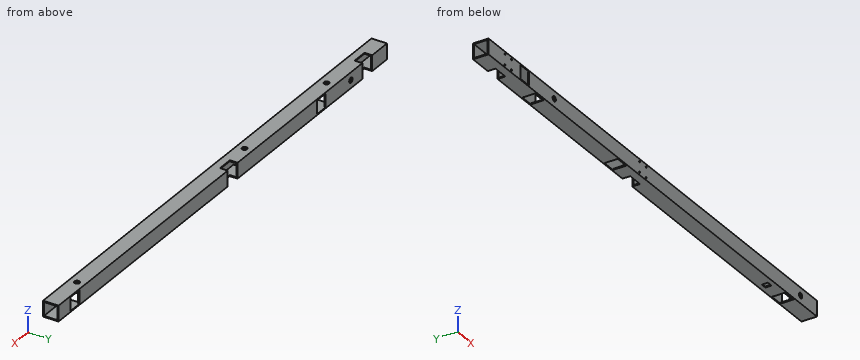
from build123d import *

# Parameters (mm, degrees)
SKETCH_2_W          = 30
SKETCH_2_H          = 30
SKETCH_2_W_2        = 26
SKETCH_2_H_2        = 26
EXTRUDE_2_DEPTH     = 1000
SKETCH_3_W          = 30
SKETCH_3_H          = 15
CUT_EXTRUDE_1_DEPTH = 30
SKETCH_4_W          = 26
SKETCH_4_H          = 26
SKETCH_4_W_2        = 11
SKETCH_4_H_2        = 12
CUT_EXTRUDE_2_DEPTH = 15
SKETCH_5_R          = 5
CUT_EXTRUDE_3_DEPTH = 15
SKETCH_6_R          = 1.5
CUT_EXTRUDE_4_DEPTH = 15
SKETCH_8_R          = 5
SKETCH_8_W          = 26
SKETCH_8_H          = 26
CUT_EXTRUDE_5_DEPTH = 15
SKETCH_9_R          = 5
SKETCH_9_W          = 26
SKETCH_9_H          = 26
CUT_EXTRUDE_6_DEPTH = 15


with BuildPart() as part:
    # 草图2 → 凸台-拉伸2 (new body)
    with BuildSketch(Plane(origin=(0, 0, 0), x_dir=(0, 0, -1), z_dir=(1, 0, 0))):
        Rectangle(SKETCH_2_W, SKETCH_2_H)
        Rectangle(SKETCH_2_W_2, SKETCH_2_H_2, mode=Mode.SUBTRACT)
    extrude(amount=EXTRUDE_2_DEPTH)

    # 草图3 → 切除-拉伸1 (cut)
    with BuildSketch(Plane(origin=(0, 0, -15), x_dir=(-1, 0, 0), z_dir=(0, 0, -1))):
        with Locations((-470, 7.5)):
            Rectangle(SKETCH_3_W, SKETCH_3_H)
        with Locations((-60, 7.5)):
            Rectangle(SKETCH_3_W, SKETCH_3_H)
    extrude(amount=-CUT_EXTRUDE_1_DEPTH, mode=Mode.SUBTRACT)

    # 草图4 → 切除-拉伸2 (cut)
    with BuildSketch(Plane(origin=(0, 0, -15), x_dir=(-1, 0, 0), z_dir=(0, 0, -1))):
        with Locations((-920, 0)):
            Rectangle(SKETCH_4_W, SKETCH_4_H)
        with Locations((-410, 0)):
            Rectangle(SKETCH_4_W, SKETCH_4_H)
        with Locations((-160, 0)):
            Rectangle(SKETCH_4_W, SKETCH_4_H)
        with Locations((-870.5, 0)):
            Rectangle(SKETCH_4_W_2, SKETCH_4_H_2)
    extrude(amount=-CUT_EXTRUDE_2_DEPTH, mode=Mode.SUBTRACT)

    # 草图5 → 切除-拉伸3 (cut)
    with BuildSketch(Plane.XY.offset(15)):
        with Locations((160, 0)):
            Circle(SKETCH_5_R)
        with Locations((410, 0)):
            Circle(SKETCH_5_R)
        with Locations((920, 0)):
            Circle(SKETCH_5_R)
    extrude(amount=-CUT_EXTRUDE_3_DEPTH, mode=Mode.SUBTRACT)

    # 草图6 → 切除-拉伸4 (cut)
    with BuildSketch(Plane.XZ.offset(15)):
        with Locations(Location((50, 10, 0), (0, 0, 270))):
            Circle(SKETCH_6_R)
        with Locations(Location((70, 10, 0), (0, 0, 270))):
            Circle(SKETCH_6_R)
        with Locations(Location((50, -10, 0), (0, 0, 270))):
            Circle(SKETCH_6_R)
        with Locations(Location((70, -10, 0), (0, 0, 270))):
            Circle(SKETCH_6_R)
        with Locations(Location((460, 10, 0), (0, 0, 270))):
            Circle(SKETCH_6_R)
        with Locations(Location((480, 10, 0), (0, 0, 270))):
            Circle(SKETCH_6_R)
        with Locations(Location((460, -10, 0), (0, 0, 270))):
            Circle(SKETCH_6_R)
        with Locations(Location((480, -10, 0), (0, 0, 270))):
            Circle(SKETCH_6_R)
    extrude(amount=-CUT_EXTRUDE_4_DEPTH, mode=Mode.SUBTRACT)

    # 草图8 → 切除-拉伸5 (cut)
    with BuildSketch(Plane(origin=(0, 15, 0), x_dir=(1, 0, 0), z_dir=(0, 1, 0))):
        with Locations(Location((110, 0, 0), (0, 0, 270))):
            Circle(SKETCH_8_R)
        with Locations((950, 0)):
            Rectangle(SKETCH_8_W, SKETCH_8_H)
        with Locations((200, 0)):
            Rectangle(SKETCH_8_W, SKETCH_8_H)
    extrude(amount=-CUT_EXTRUDE_5_DEPTH, mode=Mode.SUBTRACT)

    # 草图9 → 切除-拉伸6 (cut)
    with BuildSketch(Plane.XZ.offset(15)):
        with Locations(Location((950, 0, 0), (0, 0, 270))):
            Circle(SKETCH_9_R)
        with Locations(Location((200, 0, 0), (0, 0, 270))):
            Circle(SKETCH_9_R)
        with Locations((110, 0)):
            Rectangle(SKETCH_9_W, SKETCH_9_H)
    extrude(amount=-CUT_EXTRUDE_6_DEPTH, mode=Mode.SUBTRACT)


solid = part.part
Can you work these out from the model? Positions are in its coordinate system, mm. Give positions to 0.01 mm unless a question says otherwise; leave off trailing zeros. Order: outer loops, then holes, each group sorted by start corner. A loop starts at its lowest first (then second) coordinate and runs counter-clockwise, first axis right, second up. Notation, with made-up numbers: (62.5, 70) - (95.5, 70) arc R20 ccw to (95.5, 102) - close; hole circle Ø10 at (65.25, 12). An arc over 180 degrees is marked (long way). Write each question's results on one line, items separated by ' | '.
1) Suppose I cut it at A-A, the plane x = 375. Write out the boundary of the cut face in (y, z), then the cut area to 3 significant figures.
Final values:
outline: (-15, -15) - (15, -15) - (15, 15) - (-15, 15) - close; hole (-13, -13) - (13, -13) - (13, 13) - (-13, 13) - close | area: 224 mm^2
2) Suppose I cut it at B-B, the plane z = 0. Give the number of separate pieces and of enclosed holes in the cut face, then the cut area to 3 significant figures.
Final values:
separate pieces: 10 | enclosed holes: 0 | area: 3,660 mm^2
3) I'm going to push flat-ended pins straight in: pin 1 Ø0.6 at (x, z) = (464, -13.5) entering from +Y; pin 2 Ø8.5 at (x, z) = (118.5, -8) entering from -Y. Where does each tip first touch, or does it pass through?
Final values:
pin 1: stops at y = 0 | pin 2: stops at y = 13
4) Please list where these lines run through material, in increasing order: line 1 along Z through (x, y) = (70, -13.6); line 2 along X through (y, z) = (-14.25, -10); line 3 along Y through (x, z) = (561, -11). Write a range as [from, to].
Final values:
line 1: z = [-15, -11.5], [-8.5, 8.5], [11.5, 15] | line 2: x = [0, 48.5], [51.5, 68.5], [71.5, 97], [123, 458.5], [461.5, 478.5], [481.5, 1000] | line 3: y = [-15, -13], [13, 15]
